Design review of the part built by this model. Coordinates are the model's own, in mm. A direction names the side the tool comes from. Coordinates: 2 decimals unless noted, no trailing zeros. Loops run counter-clockwise (first coordinate to the right, second up) from the corner with the lowest first, then second, coordinate; pieces in that order, holes last. Notation, with made-up numbers: (-3.5, -7.5) - (52.5, -7.5) arc R25 ccw to (52.5, 10.5) - close; hole circle Ø7 at (-11, 29.25). An arc over 180 degrees is marked (long way). One line per question, with ' | ' between items.
from build123d import *

# Parameters (mm, degrees)
BOSS_EXTRUDE1_DEPTH = 3


with BuildPart() as part:
    # Sketch1 → Boss-Extrude1 (new body)
    with BuildSketch(Plane(origin=(0, 0, 0), x_dir=(0, 0, -1), z_dir=(1, 0, 0))):
        Polygon((-2.8, -60), (2.8, -60), (2.8, -50.4), (1.55, -50.4), (1.55, -48.2), (2.8, -48.2), (2.8, -43.2), (6, -43.2), (6, -48.2), (7.25, -48.2), (7.25, -50.4), (6, -50.4), (6, -60), (15, -60), (15, 60), (15, 71), (8.3, 71), (8.3, 65), (1.6, 65), (1.6, 55.4), (2.85, 55.4), (2.85, 53.2), (1.6, 53.2), (1.6, 48.2), (-1.6, 48.2), (-1.6, 53.2), (-2.85, 53.2), (-2.85, 55.4), (-1.6, 55.4), (-1.6, 65), (-8.3, 65), (-8.3, 71), (-15, 71), (-15, 60), (-15, 55), (-15, 50), (-18, 50), (-18, 16.6), (-15, 16.6), (-15, 6.6), (-2.4, 6.6), (-2.4, 7.85), (-0.2, 7.85), (-0.2, 6.6), (4.8, 6.6), (4.8, 3.4), (-0.2, 3.4), (-0.2, 2.15), (-2.4, 2.15), (-2.4, 3.4), (-15, 3.4), (-15, -6.6), (-18, -6.6), (-18, -50), (-15, -50), (-15, -60), (-6, -60), (-6, -50.4), (-7.25, -50.4), (-7.25, -48.2), (-6, -48.2), (-6, -43.2), (-2.8, -43.2), (-2.8, -48.2), (-1.55, -48.2), (-1.55, -50.4), (-2.8, -50.4), align=None)
    extrude(amount=BOSS_EXTRUDE1_DEPTH)


solid = part.part
Q1. Tool access review of faces 1 (the flat face through (1, -55, 2.8)), 2 (the flat face through (1, 3.4, 9)), 3 (the flat face through (1, 54, -2.85)), 4 (the flat face through (1, 60, 1.6)): name each direction out of +Z, -Z, +X, -X, +Y, -Y from which nothing blocks a thin tool from reaching the whole face with its end or side.
Returned:
face 1: +X, -X, -Y | face 2: +Z, +X, -X | face 3: +X, -X | face 4: +X, -X, +Y
Q2. For pin 1 (0.9 mm diameter, centred on x = 1.5, z = 4, fed in from -Y); pin 2 (1 mm diameter, centred on x = 1.5, z = -5, fed in from +Y); pin 3 (1.5 mm diameter, centred on x = 1, z = 17, fed in from +Y), all flat-tipped, find the tip position at first contact; note any pin that passes through.
Returned:
pin 1: stops at y = -43.2 | pin 2: stops at y = 65 | pin 3: stops at y = 50
Q3. Take a section at B-B (y = 51.5). Give the boundary of the cut face in (x, z), plus the area to 3 significant figures.
Returned:
outline: (0, -15) - (3, -15) - (3, -1.6) - (0, -1.6) - close; (0, 1.6) - (3, 1.6) - (3, 15) - (0, 15) - close | area: 80.4 mm²
Q4. Draft analysis for pull direction Z (two halves, no side actions). For faces 5 (the flat face through (1, -50, 17)), 6 (the flat face through (1, 34, 18)), 7 (the flat face through (1, -49, 7.25)), state which applies: +Z half, -Z half, draft (parallel to the pull), parting line (faces both ways), or undercut.
Returned:
face 5: draft | face 6: +Z half | face 7: undercut
Q5. To check wall thickness, follow line 1 along Y through (x, z) = (1.25, 2.5); line 2 along Z through (x, y) = (0.9, 55); line 3 along Z through (x, y) = (2.55, 2.5). State the ranges of each line that lie inside material, in increasing order.
Returned:
line 1: y = -60 to -50.4, -48.2 to 3.4, 6.6 to 53.2, 55.4 to 65 | line 2: z = -15 to -2.85, 2.85 to 15 | line 3: z = -15 to 0.2, 2.4 to 15
Q6. Take a section at A-A (z = 4). Give the boundary of the cut face in (x, y), plus the area to 3 significant figures.
Returned:
outline: (0, -43.2) - (3, -43.2) - (3, 3.4) - (0, 3.4) - close; (0, 6.6) - (3, 6.6) - (3, 65) - (0, 65) - close | area: 315 mm²
